Answer from the drawing. Dimensions are ordinates in mm from the lowest x, y and z of the part. A direction names the side the tool comes from. Coordinates: 2 decimals unless noted, no trailing zeros. Order: outer loops, then holes, each group sorted by start corner. A loop starts at its lowest first (then second) coordinate and runs counter-clockwise, first axis right, second up.
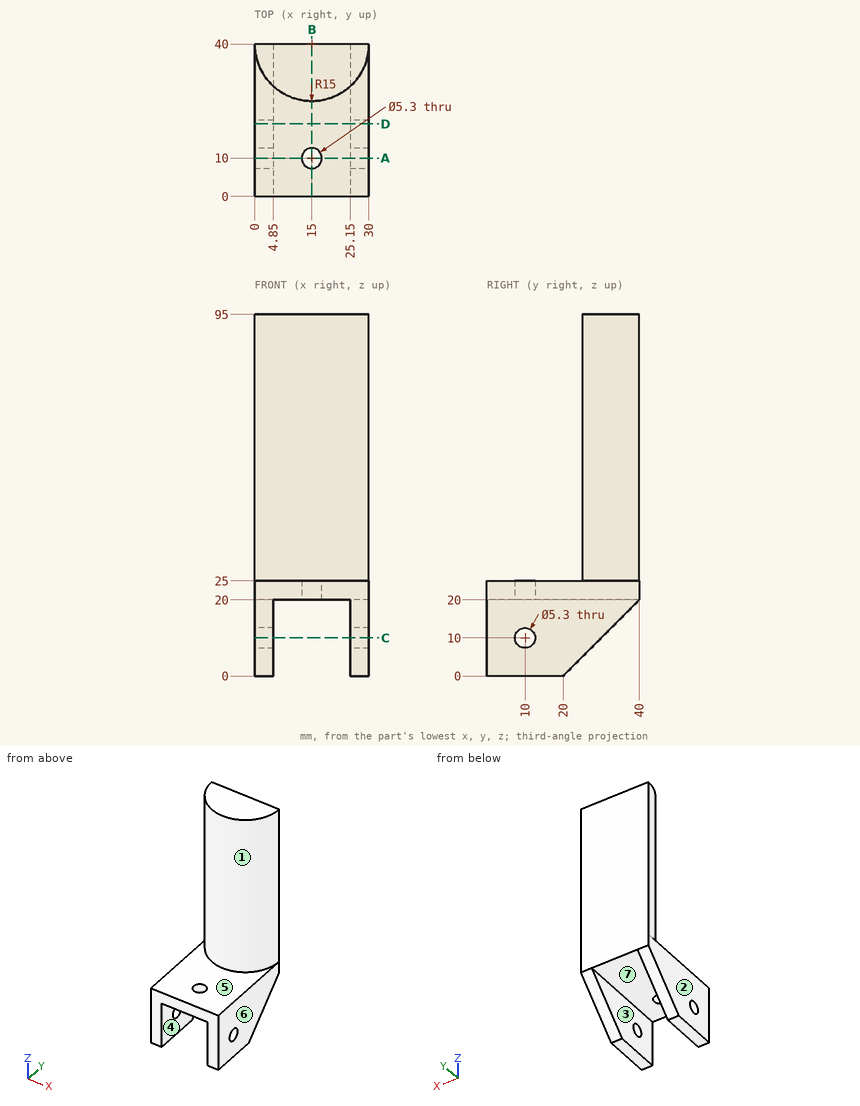
1. For the marked faces 1, 2 and 3, determine the directions among +Z, -Z, +X, -X, +Y, -Y from which every point of the face is accessible in a straight line to the end or side of a thin tool.
2. The part is cut by section B-B (x = 15). Determine the outline of the cut face in (y, z).
3. The part is cut by section D-D (y = 19). Determine the outline of the cut face in (x, z), plus the area to 3 significant figures.
4. Consider probe 1 along X at (y, z) = (30, 16.5); probe 2 along Z at (x, y) = (28.5, 10); probe 3 along Z at (x, y) = (6.75, 17.5). Determine where each line is inside the solid, lowest interval first.
5. The mould has two halves that part along X. Classify the marked faces 4, 5, 6 and 7: released by +X, released by -X, zero draft, split by the parting line, or undercut.
6. The part is cut by section A-A (y = 10). Determine the outline of the cut face in (x, z).
7. The part is cut by section C-C (z = 10). Determine the outline of the cut face in (x, y), plus the area to 3 significant figures.
8. Flat-ended cylindrical pins translate along their axes: pin 1 (16 mm diameter, centred on x = 15, y = 16, fed in from -Z); pin 2 (5 mm diameter, centred on x = 26, z = 36.5, fed in from -Y); pin 3 (3 mm diameter, centred on x = 3.5, y = 23, fed in from -Z). Find the tip coordinate at first contact, or state that the pin passes through.
Worked out:
1. face 1: +Z, -Y
1. face 2: +Z, -Z, -X, +Y, -Y
1. face 3: -Z, +Y, -Y
2. outline: (0, 20) - (7.35, 20) - (7.35, 25) - (0, 25) - close; (12.65, 20) - (40, 20) - (40, 95) - (25, 95) - (25, 25) - (12.65, 25) - close
3. outline: (0, 0) - (4.85, 0) - (4.85, 20) - (25.15, 20) - (25.15, 0) - (30, 0) - (30, 25) - (0, 25) - close
3. area: 344 mm2
4. probe 1: x = 0 to 4.85, 25.15 to 30
4. probe 2: z = 0 to 7.35, 12.65 to 25
4. probe 3: z = 20 to 25
5. face 4: undercut
5. face 5: zero draft
5. face 6: released by +X
5. face 7: undercut
6. outline: (0, 0) - (4.85, 0) - (4.85, 7.35) - (0, 7.35) - close; (0, 12.65) - (4.85, 12.65) - (4.85, 20) - (12.35, 20) - (12.35, 25) - (0, 25) - close; (17.65, 20) - (25.15, 20) - (25.15, 12.65) - (30, 12.65) - (30, 25) - (17.65, 25) - close; (25.15, 0) - (30, 0) - (30, 7.35) - (25.15, 7.35) - close
7. outline: (0, 0) - (4.85, 0) - (4.85, 7.35) - (0, 7.35) - close; (0, 12.65) - (4.85, 12.65) - (4.85, 30) - (0, 30) - close; (25.15, 0) - (30, 0) - (30, 7.35) - (25.15, 7.35) - close; (25.15, 12.65) - (30, 12.65) - (30, 30) - (25.15, 30) - close
7. area: 240 mm2
8. pin 1: stops at z = 20
8. pin 2: stops at y = 27.64
8. pin 3: stops at z = 1.5
